Drawing for the job (mm, zero at the part's lowest x, y, z). Give positions to 0.01 mm unless a question says otherwise; leave off trailing zeros. Order: outer loops, then holes, each group sorted by start corner. A loop starts at its lowest first (then second) coordinate and runs counter-clockwise, first axis right, second up. Notation, with made-up numbers: (85.25, -16) - (108.25, -16) arc R18 cw to (108.25, 9) - close; hole circle Ø7 at (40.5, 10.25). An arc over 180 degrees is marked (long way). Use a Markdown table: item, result. Add a question column.
(1) Mould opens along X. For the marked faces 1, 2, 3 and 4 say: +X half, -X half, draft (parallel to the pull), parting line (faces both ways), or undercut.
(2) Flat gauge pins, fed straight in: pin 1 (5 mm diameter, centred on y = 4, z = 6, fed in from -X); pin 2 (6 mm diameter, centred on y = 1.5, z = 24, fed in from +X); pin 3 (2 mm diameter, centred on y = 8.5, z = 35.5, fed in from +X). Where does each tip first touch, or does it go through?
(3) Slice it at B-B (z = 20.25). Write the cut outline in (x, y), then the cut area to 3 significant figures.
(4) Slice it at A-A (x = 20.25). Write the cut outline in (y, z), then the cut area to 3 significant figures.
(5) Wall check: line 1 (Z direction, x = 20.25, y = 7); line 2 (X direction, y = 5.75, z = 6.5). Give the ranges that are in metal, low to high.
(6) Slice it at C-C (y = 5). Write the cut outline in (x, z).
(7) Slice it at D-D (z = 3.5). Write the cut outline in (x, y).
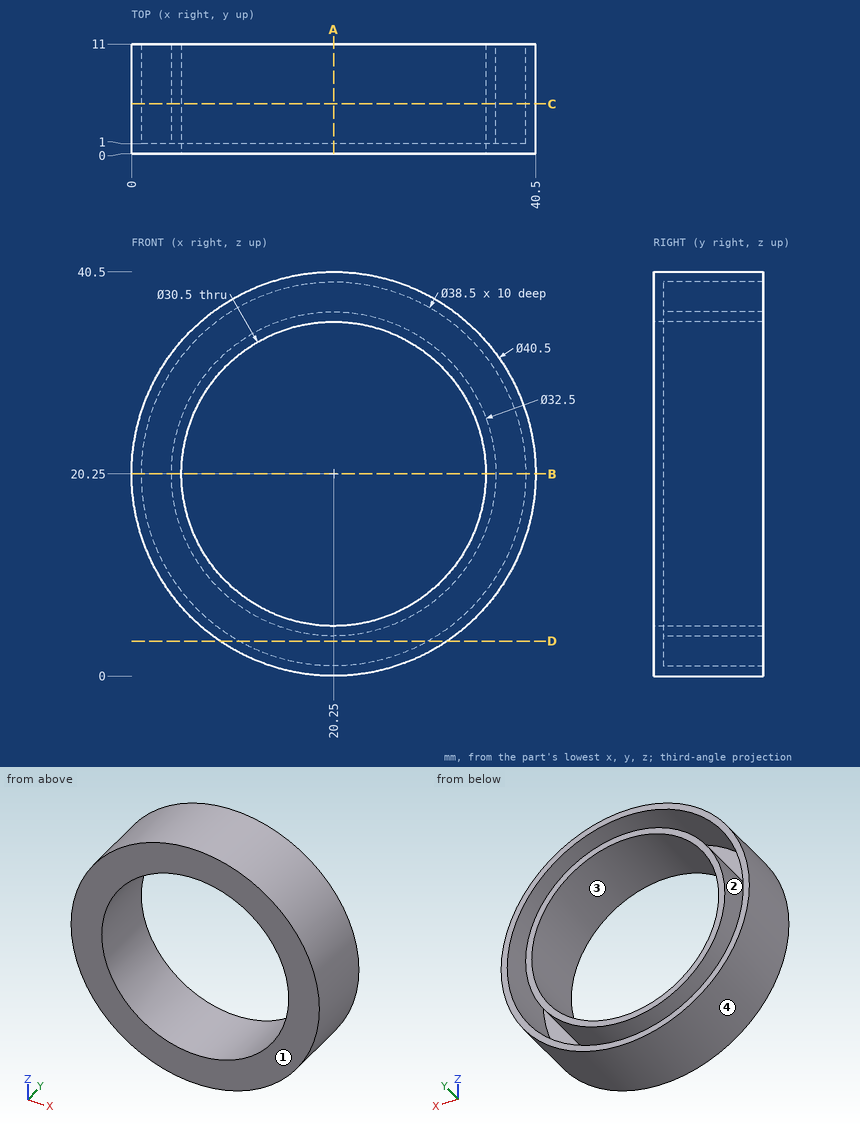
Solution:
| question | item | result |
|---|---|---|
| 1 | face 1 | draft |
| 1 | face 2 | undercut |
| 1 | face 3 | undercut |
| 1 | face 4 | parting line |
| 2 | pin 1 | x = 3.76 |
| 2 | pin 2 | x = 40.49 |
| 2 | pin 3 | x = 34.64 |
| 3 | outline | (0, 0) - (5, 0) - (5, 11) - (4, 11) - (4, 1) - (1, 1) - (1, 11) - (0, 11) - close; (35.5, 0) - (40.5, 0) - (40.5, 11) - (39.5, 11) - (39.5, 1) - (36.5, 1) - (36.5, 11) - (35.5, 11) - close |
| 3 | area | 50.0 mm2 |
| 4 | outline | (0, 0) - (11, 0) - (11, 1) - (1, 1) - (1, 4) - (11, 4) - (11, 5) - (0, 5) - close; (0, 35.5) - (11, 35.5) - (11, 36.5) - (1, 36.5) - (1, 39.5) - (11, 39.5) - (11, 40.5) - (0, 40.5) - close |
| 4 | area | 50.0 mm2 |
| 5 | line 1 | 0 to 1, 4 to 5, 35.5 to 36.5, 39.5 to 40.5 |
| 5 | line 2 | 5.38 to 6.78, 11.59 to 13.65, 26.85 to 28.91, 33.72 to 35.12 |
| 6 | outline | circle Ø40.5 at (20.25, 20.25); circle Ø32.5 at (20.25, 20.25); hole circle Ø38.5 at (20.25, 20.25); hole circle Ø30.5 at (20.25, 20.25) |
| 7 | outline | (8.87, 0) - (31.63, 0) - (31.63, 11) - (29.74, 11) - (29.74, 1) - (10.76, 1) - (10.76, 11) - (8.87, 11) - close |
